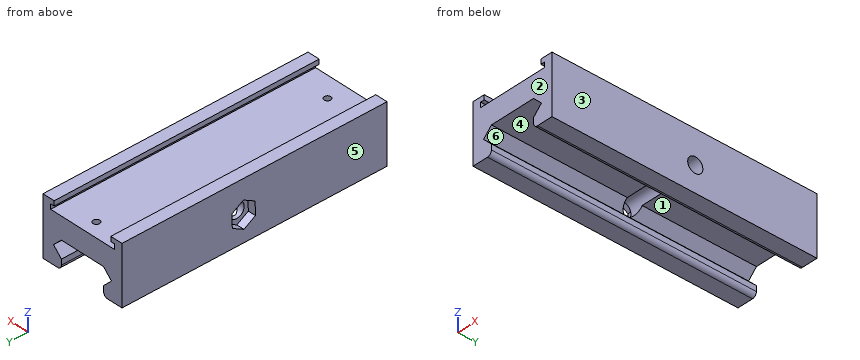
```python
from build123d import *

# Parameters (mm, degrees)
F1_DEPTH = 92.8
F3_DEPTH = 92.8
F4_R     = 1.15
F5_DEPTH = 6.6
F6_R     = 2.65
F7_DEPTH = 30
F9_DEPTH = 2.7


with BuildPart() as f1:
    # F0 (on Front) → F1 (new body)
    with BuildSketch(Plane.XZ):
        with BuildLine():
            Line((-15, 20.4), (-15, 0))
            Line((-15, 0), (-9.5, 0))
            ThreePointArc((-9.5, 0), (-8.43934, 0.43934), (-8, 1.5))
            Line((-8, 1.5), (-8, 3.4))
            Line((-8, 3.4), (-9.5, 4.9))
            Line((-9.5, 4.9), (-11, 6.4))
            Line((-11, 6.4), (-9.5, 7.9))
            Line((-9.5, 7.9), (-8, 9.4))
            Line((-8, 9.4), (0, 9.4))
            Line((0, 9.4), (8, 9.4))
            Line((8, 9.4), (11, 6.4))
            Line((11, 6.4), (8, 3.4))
            Line((8, 3.4), (8, 1.5))
            ThreePointArc((8, 1.5), (8.43934, 0.43934), (9.5, 0))
            Line((9.5, 0), (15, 0))
            Line((15, 0), (15, 20.4))
            Line((15, 20.4), (0, 20.4))
            Line((0, 20.4), (-15, 20.4))
        make_face()
    extrude(amount=F1_DEPTH)

    # F2 (on face) → F3 (cut, through all)
    with BuildSketch(Plane(origin=(0, 0, 0), x_dir=(-1, 0, 0), z_dir=(0, 1, 0))):
        Polygon((0, 20.4), (-10.75, 20.4), (-10.75, 18.75), (-12.1, 18.75), (-12.1, 17), (0, 17), (12.1, 17), (12.1, 18.75), (10.75, 18.75), (10.75, 20.4), align=None)
    extrude(amount=-F3_DEPTH, mode=Mode.SUBTRACT)

    # F4 (on face) → F5 (cut)
    with BuildSketch(Plane.XY.offset(17)):
        with Locations((0, -4.88)):
            Circle(F4_R)
        with Locations((0, -85.8)):
            Circle(F4_R)
    extrude(amount=-F5_DEPTH, mode=Mode.SUBTRACT)

    # F6 (on face) → F7 (cut)
    with BuildSketch(Plane.YZ.offset(15)):
        with Locations((-42.625, 8.9)):
            Circle(F6_R)
    extrude(amount=-F7_DEPTH, mode=Mode.SUBTRACT)

    # F8 (on face) → F9 (cut)
    with BuildSketch(Plane(origin=(-15, 0, 0), x_dir=(0, -1, 0), z_dir=(-1, 0, 0))):
        Polygon((46.628252, 11.317431), (42.533069, 13.575634), (38.529817, 11.158202), (38.621748, 6.482569), (42.716931, 4.224366), (46.720183, 6.641798), align=None)
    extrude(amount=-F9_DEPTH, mode=Mode.SUBTRACT)


solid = f1.part
```
Model file for the job. Use its own axes, mm. Face numbers are marked on the shaded views. A direction names the side the tool comes from. Coordinates: 2 decimals unless noted, no trailing zeros. Order: outer loops, then holes, each group sorted by start corner. A loop starts at its lowest first (then second) coordinate and runs counter-clockwise, first axis right, second up. Notation, with made-up numbers: (40.5, 86) - (64.5, 86) arc R14 cw to (64.5, 100) - close; hole circle Ø5 at (-17.5, 34.25). An arc over 180 degrees is marked (long way). Return JSON: item names as keys, results as strings. Group by question number.
1) Flat gauge pins, fed straight in: P1, Ø12, axis at x = -0.5, y = -45.5, coming from the +Z side; P2, Ø5, axis at x = -2.5, y = -13, coming from the -Z side; P3, Ø3, axis at x = -7.5, y = -24, coming from the -Z side. Where does each tip first touch, or does it go through?
2) Saw through at C-C, the plane y = -51. Write the cut outline in (x, z).
3) Probe line 1 (Y direction, x = 0, z = 15.5); line 2 (X direction, y = -85.8, z = 12.25); line 3 (X direction, y = -37, z = 17.5). List the from-to ranges inside material, lowest first. Write a range as from..to.
4) Saw through at A-A, the plane y = -4.88. Write the cut outline in (x, z).
5) Saw through at B-B, the plane x = 3. Write the cut outline in (y, z) (3 decimals).
6) Tool access for the marked faces 4, 5 and 6: list every direction of +Z, -Z, +X, -X, +Y, -Y with a clear straight run to the whole face (end or side of a thin tool).
7) Mould opens along X. For the marked faces 1, 2 and 3 say: released by +X, released by -X, zero draft, split by the parting line, or undercut.
Values found:
{
 "1": {"P1": "stops at z = 17", "P2": "stops at z = 9.4", "P3": "stops at z = 0.09"},
 "2": {"outline": "(-15, 0) - (-9.5, 0) arc R1.5 ccw to (-8, 1.5) - (-8, 3.4) - (-11, 6.4) - (-8, 9.4) - (8, 9.4) - (11, 6.4) - (8, 3.4) - (8, 1.5) arc R1.5 ccw to (9.5, 0) - (15, 0) - (15, 20.4) - (10.75, 20.4) - (10.75, 18.75) - (12.1, 18.75) - (12.1, 17) - (-12.1, 17) - (-12.1, 18.75) - (-10.75, 18.75) - (-10.75, 20.4) - (-15, 20.4) - close"},
 "3": {"line 1": "y = -92.8..-86.95, -84.65..-6.03, -3.73..0", "line 2": "x = -15..-1.15, 1.15..15", "line 3": "x = -15..-12.1, 12.1..15"},
 "4": {"outline": "(-15, 0) - (-9.5, 0) arc R1.5 ccw to (-8, 1.5) - (-8, 3.4) - (-11, 6.4) - (-8, 9.4) - (8, 9.4) - (11, 6.4) - (8, 3.4) - (8, 1.5) arc R1.5 ccw to (9.5, 0) - (15, 0) - (15, 20.4) - (10.75, 20.4) - (10.75, 18.75) - (12.1, 18.75) - (12.1, 17) - (1.15, 17) - (1.15, 10.4) - (-1.15, 10.4) - (-1.15, 17) - (-12.1, 17) - (-12.1, 18.75) - (-10.75, 18.75) - (-10.75, 20.4) - (-15, 20.4) - close"},
 "5": {"outline": "(-92.8, 9.4) - (-45.227, 9.4) arc R2.65 cw to (-40.023, 9.4) - (0, 9.4) - (0, 17) - (-92.8, 17) - close"},
 "6": {"face 4": "-Z, +Y, -Y", "face 5": "+Z, -Z, -X, +Y, -Y", "face 6": "+Y, -Y"},
 "7": {"face 1": "undercut", "face 2": "zero draft", "face 3": "released by +X"}
}
